```python
from build123d import *

# Parameters (mm, degrees)
SKETCH1_W           = 40
SKETCH1_H           = 10
BOSS_EXTRUDE1_DEPTH = 5
SKETCH2_W           = 4.9
SKETCH2_H           = 20
BOSS_EXTRUDE2_DEPTH = 40
CUT_EXTRUDE1_REACH  = 58.125
SKETCH3_R           = 1.6
CUT_EXTRUDE2_REACH  = 58.125
CUT_EXTRUDE3_REACH  = 58.125
CUT_EXTRUDE4_REACH  = 53.478
SKETCH6_R           = 1.6
SKETCH7_W           = 10.2
SKETCH7_H           = 3
BOSS_EXTRUDE3_DEPTH = 40
CUT_EXTRUDE5_DEPTH  = 40
SKETCH10_W          = 10.2
SKETCH10_H          = 2
BOSS_EXTRUDE4_DEPTH = 12


with BuildPart() as part:
    # Sketch1 → Boss-Extrude1 (new body)
    with BuildSketch(Plane.XY):
        Rectangle(SKETCH1_W, SKETCH1_H)
    extrude(amount=BOSS_EXTRUDE1_DEPTH)

    # Sketch2 → Boss-Extrude2 (add)
    with BuildSketch(Plane.XY.offset(5)):
        with Locations((7.55, 5)):
            Rectangle(SKETCH2_W, SKETCH2_H)
        with Locations((-7.55, 5)):
            Rectangle(SKETCH2_W, SKETCH2_H)
    extrude(amount=BOSS_EXTRUDE2_DEPTH)

    # Cut-Extrude1: up to this face of the body (flat: up to its plane)
    cut_extrude1_end = Plane(part.part.faces().sort_by_distance((10, 5, 25))[0])
    # Sketch3 → Cut-Extrude1 (cut, up to the picked face)
    with BuildSketch(Plane.ZY.offset(10), mode=Mode.PRIVATE) as cut_extrude1_sk1:
        with Locations((40, 10)):
            Circle(SKETCH3_R)
    cut_extrude1_tool1 = split(extrude(cut_extrude1_sk1.sketch, amount=-CUT_EXTRUDE1_REACH, mode=Mode.PRIVATE), bisect_by=cut_extrude1_end, keep=Keep.BOTH, mode=Mode.PRIVATE)
    # Sketch3 → Cut-Extrude1 (cut, up to the picked face)
    with BuildSketch(Plane.ZY.offset(10), mode=Mode.PRIVATE) as cut_extrude1_sk2:
        with Locations((25, 10)):
            Circle(SKETCH3_R)
    cut_extrude1_tool2 = split(extrude(cut_extrude1_sk2.sketch, amount=-CUT_EXTRUDE1_REACH, mode=Mode.PRIVATE), bisect_by=cut_extrude1_end, keep=Keep.BOTH, mode=Mode.PRIVATE)
    add(cut_extrude1_tool1.solids().sort_by(Axis((-10, 10, 40), (1, 0, 0)))[0], mode=Mode.SUBTRACT)
    add(cut_extrude1_tool2.solids().sort_by(Axis((-10, 10, 25), (1, 0, 0)))[0], mode=Mode.SUBTRACT)

    # Cut-Extrude2: up to this face of the body (flat: up to its plane)
    cut_extrude2_end = Plane(part.part.faces().sort_by_distance((10, 4.897406266, 24.846109398))[0])
    # Sketch4 → Cut-Extrude2 (cut, up to the picked face)
    with BuildSketch(Plane.ZY.offset(10), mode=Mode.PRIVATE) as cut_extrude2_sk1:
        Polygon((5, 5), (20, 15), (5, 15), align=None)
    cut_extrude2_tool1 = split(extrude(cut_extrude2_sk1.sketch, amount=-CUT_EXTRUDE2_REACH, mode=Mode.PRIVATE), bisect_by=cut_extrude2_end, keep=Keep.BOTH, mode=Mode.PRIVATE)
    add(cut_extrude2_tool1.solids().sort_by(Axis((-10, 11.666667, 10), (1, 0, 0)))[0], mode=Mode.SUBTRACT)

    # Cut-Extrude3: up to this face of the body (flat: up to its plane)
    cut_extrude3_end = Plane(part.part.faces().sort_by_distance((10, 4.181249184, 26.416760511))[0])
    # Sketch5 → Cut-Extrude3 (cut, up to the picked face)
    with BuildSketch(Plane.ZY.offset(10), mode=Mode.PRIVATE) as cut_extrude3_sk1:
        Polygon((45, 5), (5, -5), (45, -5), align=None)
    cut_extrude3_tool1 = split(extrude(cut_extrude3_sk1.sketch, amount=-CUT_EXTRUDE3_REACH, mode=Mode.PRIVATE), bisect_by=cut_extrude3_end, keep=Keep.BOTH, mode=Mode.PRIVATE)
    add(cut_extrude3_tool1.solids().sort_by(Axis((-10, -1.666667, 31.666667), (1, 0, 0)))[0], mode=Mode.SUBTRACT)

    # Sketch6 → Cut-Extrude4 (cut, up to next)
    with BuildSketch(Plane(origin=(0, 0, 0), x_dir=(-1, 0, 0), z_dir=(0, 0, -1)), mode=Mode.PRIVATE) as cut_extrude4_sk1:
        with Locations((-15, 0)):
            Circle(SKETCH6_R)
    cut_extrude4_tool1 = extrude(cut_extrude4_sk1.sketch, amount=-CUT_EXTRUDE4_REACH, mode=Mode.PRIVATE) & part.part
    # Sketch6 → Cut-Extrude4 (cut, up to next)
    with BuildSketch(Plane(origin=(0, 0, 0), x_dir=(-1, 0, 0), z_dir=(0, 0, -1)), mode=Mode.PRIVATE) as cut_extrude4_sk2:
        with Locations(Location((15, 0, 0), (0, 0, 180))):
            Circle(SKETCH6_R)
    cut_extrude4_tool2 = extrude(cut_extrude4_sk2.sketch, amount=-CUT_EXTRUDE4_REACH, mode=Mode.PRIVATE) & part.part
    add(cut_extrude4_tool1.solids().sort_by_distance((15, 0, 0))[0], mode=Mode.SUBTRACT)
    add(cut_extrude4_tool2.solids().sort_by_distance((-15, 0, 0))[0], mode=Mode.SUBTRACT)

    # Sketch7 → Boss-Extrude3 (add)
    with BuildSketch(Plane.XY.offset(5)):
        with Locations((0, -3.5)):
            Rectangle(SKETCH7_W, SKETCH7_H)
    extrude(amount=BOSS_EXTRUDE3_DEPTH)

    # Sketch8 → Cut-Extrude5 (cut)
    with BuildSketch(Plane.ZY.offset(5.1)):
        Polygon((5, -5), (25, 0), (45, 0), (45, -5), align=None)
    extrude(amount=-CUT_EXTRUDE5_DEPTH, mode=Mode.SUBTRACT)

    # Sketch10 → Boss-Extrude4 (add)
    with BuildSketch(Plane.XY.offset(5)):
        with Locations((0, -1)):
            Rectangle(SKETCH10_W, SKETCH10_H)
    extrude(amount=BOSS_EXTRUDE4_DEPTH)


solid = part.part
```
For this review, take the finished solid that the model builds, in its own axes (mm). A direction names the side the tool comes from. Coordinates: 2 decimals unless noted, no trailing zeros. Write each loop counter-clockwise with the first axis right and the second up, starting at its lowest first coordinate (ties: lowest second). Pieces come first, ordered by that corner, then holes. Notation, with made-up numbers: (80, 62) - (114, 62) arc R21 ccw to (114, 89) - close; hole circle Ø11 at (3, 83.5). An arc over 180 degrees is marked (long way). Put each result on its own line as item: value.
1. Add section D-D, the plane x = -3.5. Give the boundary of the cut face in (y, z), then the cut area to 3 significant figures.
Values found:
outline: (-5, 0) - (5, 0) - (5, 5) - (0, 5) - (0, 17) - (-2, 17) - (-5, 5) - close
area: 92.0 mm²
2. Add section C-C, the plane y = 10. Give the boundary of the cut face in (x, z), then the cut area to 3 significant figures.
Values found:
outline: (-10, 12.5) - (-5.1, 12.5) - (-5.1, 23.4) - (-10, 23.4) - close; (-10, 26.6) - (-5.1, 26.6) - (-5.1, 38.4) - (-10, 38.4) - close; (-10, 41.6) - (-5.1, 41.6) - (-5.1, 45) - (-10, 45) - close; (5.1, 12.5) - (10, 12.5) - (10, 23.4) - (5.1, 23.4) - close; (5.1, 26.6) - (10, 26.6) - (10, 38.4) - (5.1, 38.4) - close; (5.1, 41.6) - (10, 41.6) - (10, 45) - (5.1, 45) - close
area: 256 mm²
3. Mouldability with a two-part tool opening along X and no side actions: class faces 5 (the flat face through (-0.14, -2.152, 16.391)), 6 (the flat face through (-10, 7, 25)), 7 (the flat face through (0, -1, 17)) as released by +X, released by -X, zero draft, split by the parting line, or undercut.
Values found:
face 5: zero draft
face 6: released by -X
face 7: undercut
4. For pin 1 (5 mm diameter, centred on x = -8.5, z = 6.5, fed in from +Y); pin 2 (5 mm diameter, centred on x = 15, y = 0, fed in from +Z); pin 3 (5 mm diameter, centred on x = 1.5, z = 18, fed in from -Y) (3 decimals); pin 4 (5 mm diameter, centred on x = 13, y = 12.5, fed in from -Z), all flat-tipped, find the tip position at first contact; note any pin that passes through.
Values found:
pin 1: y = 7.67
pin 2: z = 5
pin 3: y = -2.375
pin 4: through
5. Add section A-A, the plane y = 6.5. Give the boundary of the cut face in (x, z).
Values found:
outline: (-10, 7.25) - (-5.1, 7.25) - (-5.1, 45) - (-10, 45) - close; (5.1, 7.25) - (10, 7.25) - (10, 45) - (5.1, 45) - close
6. Machinability: for faces 1 (the flat face through (0, 3, 5)), 2 (the flat face through (0, 5, 2)), 3 (the flat face through (0, 0, 0)), 4 (the flat face through (10, 7, 25)), which of the approach directions +Z, -Z, +X, -X, +Y, -Y give a long, thin tool a straight path to every point of the face, cutting with its end or side? Answer none if there is none.
Values found:
face 1: +Z, +Y
face 2: -Z, +X, -X, +Y
face 3: -Z, +X, -X, +Y, -Y
face 4: +Z, +X, +Y, -Y
7. Wall thickness on probe 1 along X at (y, z) = (11.75, 38); probe 2 along Y at (x, z) = (8, 25); probe 3 along Z at (x, y) = (-6, 8.75) (3 decimals): over which ranges is each line inside the solid? List them lowest first.
Values found:
probe 1: -10 to -5.1, 5.1 to 10
probe 2: 0 to 8.4, 11.6 to 15
probe 3: 10.625 to 24.001, 25.999 to 39.001, 40.999 to 45
8. Add section B-B, the plane z = 37. Give the boundary of the cut face in (x, y).
Values found:
outline: (-10, 3) - (-5.1, 3) - (-5.1, 15) - (-10, 15) - close; (5.1, 3) - (10, 3) - (10, 15) - (5.1, 15) - close
